Here's how the part is built. I have some questions about the finished solid (model axes, mm). Face numbers are marked on the shaded views. A direction names the side the tool comes from. Coordinates: 2 decimals unless noted, no trailing zeros. Loops run counter-clockwise (first coordinate to the right, second up) from the corner with the lowest first, then second, coordinate; pieces in that order, holes last. Notation, with made-up numbers: M 87.25,-32.5 L 105.25,-32.5 A14 ccw 105.25,-18.5 Z; hole C -32,36 d7. An arc over 180 degrees is marked long. Use one line per item in the form item = value. Start each with the question number.
(1) Will these pins go through, and if not, where does the flat tip stop? P1, Ø0.8, axis at y = 8.5, z = 0, coming from the -X side; P2, Ø4, axis at x = -40, z = -4.5, coming from the -Y side; P3, Ø6, axis at x = -14.5, y = 16.5, coming from the -Z side.
(2) Imagine slicing it at A-A, the plane z = -3. Please give me the cut outline in (x, y), and give its area (3 significant figures).
(3) Imagine slicing it at C-C, the plane x = -11. Please give me the cut outline in (y, z), and give its area (3 significant figures).
(4) Imagine slicing it at D-D, the plane x = 19. Please give me the cut outline in (y, z).
(5) On a 3-axis mill with a long thin cutter (end or side, diameter ignored), from which of +Z, -Z, +X, -X, +Y, -Y can I reach the whole of each face in a straight line? I mean the marked faces 1 and 2. Say none if no direction works.
(6) Please list where these lines run through material, in increasing order: L1, parallel to X at y = 42.5, z = -1 (3 decimals); L2, parallel to Y at x = 10.5, z = 0.75; L3, parallel to X at y = 3, z = -0.75.
(7) Imagine slicing it at B-B, the plane y = 4.5. Please give me the cut outline in (x, z), and give its area (3 significant figures).
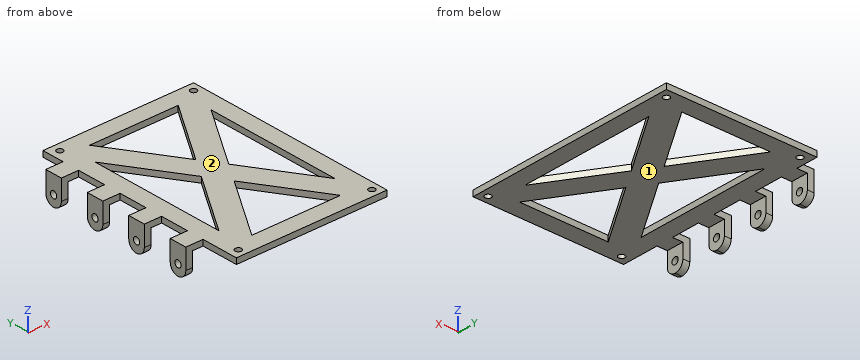
```python
from build123d import *

# Parameters (mm, degrees)
SKETCH1_W                = 90
SKETCH1_H                = 100
BOSS_EXTRUDE1_DEPTH      = 1.25
CUT_EXTRUDE2_DEPTH       = 68.314560089
CUT_EXTRUDE2_DEPTH_BACK  = 68.314560089
SKETCH3_W                = 120.524160128
SKETCH3_H                = 121.100830751
SKETCH3_W_2              = 90
SKETCH3_H_2              = 100
BOSS_EXTRUDE2_DEPTH      = 10
BOSS_EXTRUDE2_DEPTH_BACK = 1
SKETCH4_W                = 3
SKETCH4_H                = 7.5
CUT_EXTRUDE4_DEPTH       = 85.83221669
CUT_EXTRUDE4_DEPTH_BACK  = 85.83221669
SKETCH6_R                = 1.5
HOLDER_SCREW_DEPTH       = 65.47473997
HOLDER_SCREW_DEPTH_BACK  = 65.47473997
SKETCH11_R               = 1.375


with BuildPart() as part:
    # Sketch1 → Boss-Extrude1 (new, symmetric)
    with BuildSketch(Plane.XY):
        Rectangle(SKETCH1_W, SKETCH1_H)
    extrude(amount=BOSS_EXTRUDE1_DEPTH, both=True)

    # Sketch3 → Cut-Extrude2 (cut, two sides: drawn at the far end of the back side and taken through both)
    # profile 1 of 6: a face of its own
    with BuildSketch(Plane(origin=(0, 0, -1.25), x_dir=(-1, 0, 0), z_dir=(0, 0, -1)).offset(-CUT_EXTRUDE2_DEPTH_BACK)):
        with Locations((6.594005418, 0.079563665)):
            Rectangle(SKETCH3_W, SKETCH3_H)
        Rectangle(SKETCH3_W_2, SKETCH3_H_2, mode=Mode.SUBTRACT)
    # profile 2 of 6: a face of its own
    with BuildSketch(Plane(origin=(0, 0, -1.25), x_dir=(-1, 0, 0), z_dir=(0, 0, -1)).offset(-CUT_EXTRUDE2_DEPTH_BACK)):
        Rectangle(SKETCH3_W_2, SKETCH3_H_2)
        Polygon((42.616130373, -30.674442955), (35.116130373, -30.674442955), (35.116130373, -33.902086325), (35.116130373, -46.739785261), (-30.279040864, -46.739785261), (-30.279040864, 46.489928229), (35.116130373, 46.489928229), (35.116130373, 36.825557045), (42.616130373, 36.825557045), (42.616130373, 29.325557045), (35.116130373, 29.325557045), (35.116130373, 16.825557045), (42.616130373, 16.825557045), (42.616130373, 9.325557045), (35.116130373, 9.325557045), (35.116130373, -3.174442955), (42.616130373, -3.174442955), (42.616130373, -10.674442955), (35.116130373, -10.674442955), (35.116130373, -23.174442955), (42.616130373, -23.174442955), align=None, mode=Mode.SUBTRACT)
    # profile 3 of 6: a face of its own
    with BuildSketch(Plane(origin=(0, 0, -1.25), x_dir=(-1, 0, 0), z_dir=(0, 0, -1)).offset(-CUT_EXTRUDE2_DEPTH_BACK)):
        Polygon((-16.831379802, 38.989928229), (2.418544754, 9.1077779), (21.668469311, 38.989928229), align=None)
    # profile 4 of 6: a face of its own
    with BuildSketch(Plane(origin=(0, 0, -1.25), x_dir=(-1, 0, 0), z_dir=(0, 0, -1)).offset(-CUT_EXTRUDE2_DEPTH_BACK)):
        Polygon((-22.779040864, 29.757221813), (-22.779040864, -30.007078845), (-3.529116308, -0.124928516), align=None)
    # profile 5 of 6: a face of its own
    with BuildSketch(Plane(origin=(0, 0, -1.25), x_dir=(-1, 0, 0), z_dir=(0, 0, -1)).offset(-CUT_EXTRUDE2_DEPTH_BACK)):
        Polygon((2.418544754, -9.357634932), (21.668469311, -39.239785261), (-16.831379802, -39.239785261), align=None)
    # profile 6 of 6: a face of its own
    with BuildSketch(Plane(origin=(0, 0, -1.25), x_dir=(-1, 0, 0), z_dir=(0, 0, -1)).offset(-CUT_EXTRUDE2_DEPTH_BACK)):
        Polygon((8.366205816, -0.124928516), (27.616130373, 29.757221813), (27.616130373, -30.007078845), align=None)
    extrude(amount=CUT_EXTRUDE2_DEPTH + CUT_EXTRUDE2_DEPTH_BACK, mode=Mode.SUBTRACT)

    # Sketch4 → Boss-Extrude2 (add, two sides: drawn at the far end of the back side and taken through both)
    with BuildSketch(Plane(origin=(0, 0, -1.25), x_dir=(-1, 0, 0), z_dir=(0, 0, -1)).offset(-BOSS_EXTRUDE2_DEPTH_BACK)):
        with Locations((41.116130373, 33.075557045)):
            Rectangle(SKETCH4_W, SKETCH4_H)
        with Locations((41.116130373, 13.075557045)):
            Rectangle(SKETCH4_W, SKETCH4_H)
        with Locations((41.116130373, -6.924442955)):
            Rectangle(SKETCH4_W, SKETCH4_H)
        with Locations((41.116130373, -26.924442955)):
            Rectangle(SKETCH4_W, SKETCH4_H)
    extrude(amount=BOSS_EXTRUDE2_DEPTH + BOSS_EXTRUDE2_DEPTH_BACK)

    # Sketch6 → Cut-Extrude4 (cut, two sides: drawn at the far end of the back side and taken through both)
    with BuildSketch(Plane(origin=(-39.616130373, 0, 0), x_dir=(0, 0, -1), z_dir=(1, 0, 0)).offset(-CUT_EXTRUDE4_DEPTH_BACK)):
        with Locations((6.568537773, 33.075557045)):
            Circle(SKETCH6_R)
        with BuildLine():
            Line((11.25, 33.075557045), (11.25, 36.825557045))
            Line((11.25, 36.825557045), (7.5, 36.825557045))
            ThreePointArc((7.5, 36.825557045), (10.151650429, 35.727207475), (11.25, 33.075557045))
        make_face()
        with BuildLine():
            Line((11.25, 29.325557045), (11.25, 33.075557045))
            ThreePointArc((11.25, 33.075557045), (10.151650429, 30.423906616), (7.5, 29.325557045))
            Line((7.5, 29.325557045), (11.25, 29.325557045))
        make_face()
        with Locations((6.568537773, 13.075557045)):
            Circle(SKETCH6_R)
        with BuildLine():
            Line((11.25, 9.325557045), (11.25, 13.075557045))
            ThreePointArc((11.25, 13.075557045), (10.151650429, 10.423906616), (7.5, 9.325557045))
            Line((7.5, 9.325557045), (11.25, 9.325557045))
        make_face()
        with BuildLine():
            Line((11.25, 13.075557045), (11.25, 16.825557045))
            Line((11.25, 16.825557045), (7.5, 16.825557045))
            ThreePointArc((7.5, 16.825557045), (10.151650429, 15.727207475), (11.25, 13.075557045))
        make_face()
        with BuildLine():
            Line((11.25, -6.924442955), (11.25, -3.174442955))
            Line((11.25, -3.174442955), (7.5, -3.174442955))
            ThreePointArc((7.5, -3.174442955), (10.151650429, -4.272792525), (11.25, -6.924442955))
        make_face()
        with Locations((6.568537773, -6.924442955)):
            Circle(SKETCH6_R)
        with BuildLine():
            Line((11.25, -10.674442955), (11.25, -6.924442955))
            ThreePointArc((11.25, -6.924442955), (10.151650429, -9.576093384), (7.5, -10.674442955))
            Line((7.5, -10.674442955), (11.25, -10.674442955))
        make_face()
        with BuildLine():
            Line((11.25, -30.674442955), (11.25, -26.924442971))
            ThreePointArc((11.25, -26.924442971), (10.151650424, -29.57609339), (7.5, -30.674442955))
            Line((7.5, -30.674442955), (11.25, -30.674442955))
        make_face()
        with Locations((6.568537773, -26.924442955)):
            Circle(SKETCH6_R)
        with BuildLine():
            Line((11.25, -26.924442971), (11.25, -23.174442955))
            Line((11.25, -23.174442955), (7.5, -23.174442955))
            ThreePointArc((7.5, -23.174442955), (10.151650435, -24.272792531), (11.25, -26.924442971))
        make_face()
    extrude(amount=CUT_EXTRUDE4_DEPTH + CUT_EXTRUDE4_DEPTH_BACK, mode=Mode.SUBTRACT)

    # Sketch11 → Holder_Screw (cut, two sides: drawn at the far end of the back side and taken through both)
    with BuildSketch(Plane.XY.offset(1.25).offset(-HOLDER_SCREW_DEPTH_BACK)):
        with Locations(Location((-31.1419152, 42.7222856, 0), (0, 0, 180))):
            Circle(SKETCH11_R)
        with Locations(Location((26.8580848, 42.7222856, 0), (0, 0, 180))):
            Circle(SKETCH11_R)
        with Locations(Location((26.8580848, -43.2777144, 0), (0, 0, 180))):
            Circle(SKETCH11_R)
        with Locations(Location((-31.1419152, -43.2777144, 0), (0, 0, 180))):
            Circle(SKETCH11_R)
    extrude(amount=HOLDER_SCREW_DEPTH + HOLDER_SCREW_DEPTH_BACK, mode=Mode.SUBTRACT)


solid = part.part
```
Answer:
q1.P1 = -35.12
q1.P2 = -30.67
q1.P3 = -1.25
q2.outline = M -42.62,-30.67 L -39.62,-30.67 L -39.62,-23.17 L -42.62,-23.17 Z; M -42.62,-10.67 L -39.62,-10.67 L -39.62,-3.17 L -42.62,-3.17 Z; M -42.62,9.33 L -39.62,9.33 L -39.62,16.83 L -42.62,16.83 Z; M -42.62,29.33 L -39.62,29.33 L -39.62,36.83 L -42.62,36.83 Z
q2.area = 90.0 mm²
q3.outline = M -46.74,-1.25 L -39.24,-1.25 L -39.24,1.25 L -46.74,1.25 Z; M -22.68,-1.25 L -4.21,-1.25 L -4.21,1.25 L -22.68,1.25 Z; M 3.96,-1.25 L 22.43,-1.25 L 22.43,1.25 L 3.96,1.25 Z; M 38.99,-1.25 L 46.49,-1.25 L 46.49,1.25 L 38.99,1.25 Z
q3.area = 130 mm²
q4.outline = M -46.74,-1.25 L -24.14,-1.25 L -24.14,1.25 L -46.74,1.25 Z; M 23.89,-1.25 L 46.49,-1.25 L 46.49,1.25 L 23.89,1.25 Z
q5.face_1 = -Z, +X, +Y, -Y
q5.face_2 = +Z, +X, -X, +Y, -Y
q6.L1 = -35.116 to -32.499, -29.785 to 25.501, 28.215 to 30.279
q6.L2 = -46.74 to -39.24, -29.41 to -10.95, 10.7 to 29.16, 38.99 to 46.49
q6.L3 = -35.12 to -27.62, -10.38 to 5.54, 22.78 to 30.28
q7.outline = M -35.12,-1.25 L -27.62,-1.25 L -27.62,1.25 L -35.12,1.25 Z; M -11.35,-1.25 L 6.51,-1.25 L 6.51,1.25 L -11.35,1.25 Z; M 22.78,-1.25 L 30.28,-1.25 L 30.28,1.25 L 22.78,1.25 Z
q7.area = 82.1 mm²
